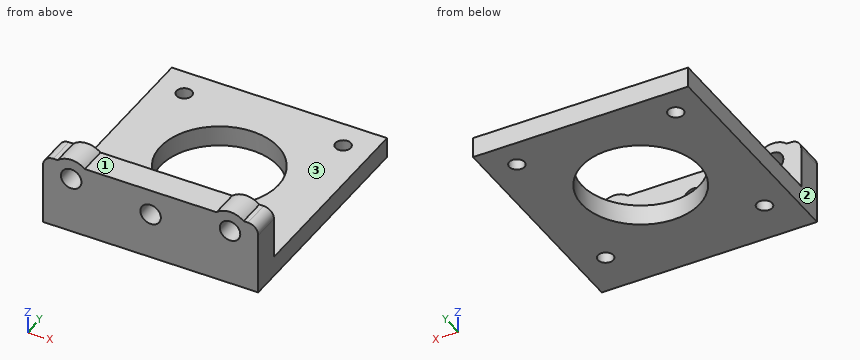
Autodesk Inventor part; units mm, degrees
ref_plane "YZ Plane" through (0, 0, 0) normal (1, 0, 0) x (0, 1, 0)
ref_plane "XZ Plane" through (0, 0, 0) normal (0, 1, 0) x (-1, 0, 0)
ref_plane "XY Plane" through (0, 0, 0) normal (0, 0, 1) x (1, 0, 0)
sketch "Sketch1" plane through (0, 0, 0) normal (0, 0, 1) x (1, 0, 0)
  circle A0 centre (0, 0) radius 11.5
  circle A1 centre (-15.5, 15.5) radius 1.5
  circle A2 centre (-15.5, -15.5) radius 1.5
  circle A3 centre (15.5, 15.5) radius 1.5
  circle A4 centre (15.5, -15.5) radius 1.5
  line L0 (-21, -24) -> (21, -24)
  line L1 (0, 20) -> (4.5462, 20) construction
  line L2 (-21, 21) -> (-1, 21)
  line L3 (1, 21) -> (21, 21)
  line L4 (-21, 21) -> (-21, 5.9161)
  line L5 (-21, -5.9161) -> (-21, -24)
  line L6 (21, 21) -> (21, 5.9161)
  line L7 (21, -5.9161) -> (21, -24)
  line L8 (-1.865, 21) -> (1.6498, 21)
  line L9 (-21, 8.451) -> (-21, -8.8551)
  line L10 (21, 10.9387) -> (21, -8.8551)
  dimension "d0" = 23
  dimension "d1" = 3
  dimension "d2" = 3
  dimension "d3" = 24
  dimension "d5" = 8.5
extrude "Extrusion1" add sketch "Sketch1" along normal blind 4
sketch "Sketch2" plane through (0, 0, 4) normal (0, 0, 1) x (1, 0, 0)
  line L0 (-21, -24) -> (21, -24)
  line L1 (21, -24) -> (21, 21)
  line L2 (-21, -24) -> (21, -24)
  line L3 (21, -24) -> (21, -18.5)
  line L4 (21, -18.5) -> (-21, -18.5)
  line L5 (-21, -18.5) -> (-21, -24)
  dimension "d9" = 5.5
extrude "Extrusion2" add sketch "Sketch2" along normal blind 10
sketch "Sketch3" plane through (-21, -24, 0) normal (0, -1, 0) x (1, 0, 0)
  line L0 (42, 0) -> (42, 14)
  line L1 (0, 0) -> (0, 14)
  circle A0 centre (5.5, 11) radius 2
  circle A1 centre (36.5, 11) radius 2
  line L2 (0, 4) -> (42, 4)
  circle A2 centre (21, 9) radius 2
  line L3 (0, 14) -> (42, 14)
  point P0 (21, 0)
  dimension "d12" = 4
  dimension "d13" = 4
  dimension "d16" = 5.5
  dimension "d17" = 5.5
  dimension "d18" = 7
  dimension "d19" = 7
  dimension "d27" = 4
  dimension "d28" = 5
sketch "Sketch4" plane through (-21, -24, 0) normal (0, -1, 0) x (1, 0, 0)
  circle A0 centre (5.5, 11) radius 2
  circle A1 centre (36.5, 11) radius 2
  arc A2 (8.1458, 14) -> (2.8542, 14) centre (5.5, 11) ccw
  arc A3 (39.1458, 14) -> (33.8542, 14) centre (36.5, 11) ccw
  line L0 (42, 14) -> (0, 14)
  line L1 (2.8542, 14) -> (8.1458, 14)
  line L2 (33.8542, 14) -> (39.1458, 14)
  point P0 (21, 0)
  dimension "d22" = 8
  dimension "d23" = 8
extrude "Extrusion4" add sketch "Sketch4" against normal blind 5.5 contours L0 A2 | A3 L0
fillet "Fillet1" radius 2 2 edges at (-21, -21.25, 14) (21, -21.25, 14)
extrude "Extrusion5" cut sketch "Sketch3" against normal blind 5.5 contours A0 | A1 | A2
properties part number "StepperMotorPlate" material "PPS Plastic"
Work out the finished part from the listing and answer in its coordinate system (mm). Face numbers are marked on the shaded views. A direction names the side the tool comes from. Round coordinates to 2 decimals unless told otherwise and drop trailing zeros. Write each loop counter-clockwise with the first axis right and the second up, starting at its lowest first coordinate (ties: lowest second). Pieces come first, ordered by that corner, then holes.
1) A tool of negligible diameter and unlimited length cuts with its end or side. For the marked faces 1, 2 and 3, from which of +Z, -Z, +X, -X, +Y, -Y can it reach the whole face along a straight path? Write none if from no direction.
2) Given pin 1 Ø2 at (x, y) = (-6.5, -9) entering from +Z; pin 2 Ø1.5 at (x, z) = (11.5, 6) entering from +Y; pin 3 Ø6 at (x, y) = (0, -22.5) entering from +Z, each flat-ended and moving along its own axis, determine where each tip first touches the part or whether it passes through.
3) Straight lines are drawn through the part: line 1 (Y direction, x = -15.5, z = 1.1); line 2 (Z direction, x = 0, y = -19.75); line 3 (Z direction, x = -15.5, y = -22.4). For each, find the intervals that lie inside material, in ascending order.
4) A cutting plane is placed at D-D (y = 15.5). Give the vertices of the cut face in (x, z).
5) A cutting plane is placed at B-B (z = 2.5). Give the vertices of the cut face in (x, y), plus the area to 3 significant figures.
6) A cutting plane is placed at A-A (y = 0). Give the vertices of the cut face in (x, z).
7) A cutting plane is placed at C-C (x = -15.5). Give the vertices of the cut face in (y, z).
Completed:
1. face 1: +Z, +Y, -Y
1. face 2: +Z, -Z, -X, +Y, -Y
1. face 3: +Z, +X, -X, +Y
2. pin 1: stops at z = 4
2. pin 2: stops at y = -18.5
2. pin 3: stops at z = 14
3. line 1: y = -24 to -17, -14 to 14, 17 to 21
3. line 2: z = 0 to 7, 11 to 14
3. line 3: z = 0 to 9, 13 to 15
4. outline: (-21, 0) - (-17, 0) - (-17, 4) - (-21, 4) - close; (-14, 0) - (14, 0) - (14, 4) - (-14, 4) - close; (17, 0) - (21, 0) - (21, 4) - (17, 4) - close
5. outline: (-21, -24) - (21, -24) - (21, 21) - (-21, 21) - close; hole circle Ø3 at (-15.5, -15.5); hole circle Ø3 at (-15.5, 15.5); hole circle Ø23 at (0, 0); hole circle Ø3 at (15.5, -15.5); hole circle Ø3 at (15.5, 15.5)
5. area: 1,450 mm2
6. outline: (-21, 0) - (-11.5, 0) - (-11.5, 4) - (-21, 4) - close; (11.5, 0) - (21, 0) - (21, 4) - (11.5, 4) - close
7. outline: (-24, 0) - (-17, 0) - (-17, 4) - (-18.5, 4) - (-18.5, 9) - (-24, 9) - close; (-24, 13) - (-18.5, 13) - (-18.5, 15) - (-24, 15) - close; (-14, 0) - (14, 0) - (14, 4) - (-14, 4) - close; (17, 0) - (21, 0) - (21, 4) - (17, 4) - close
